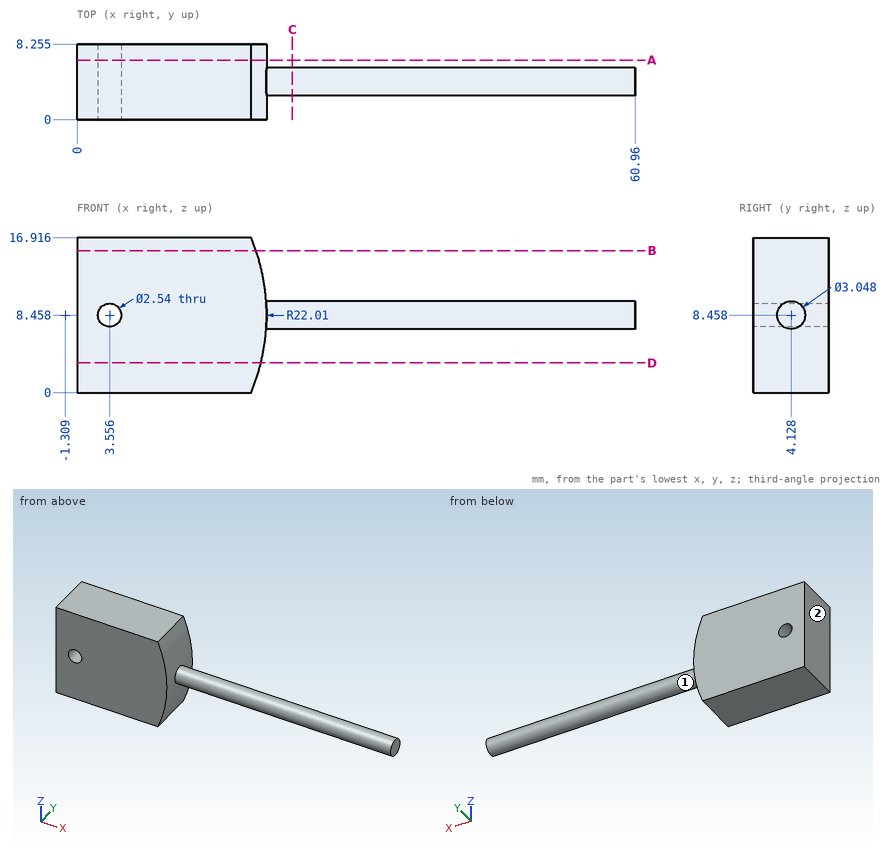
Could you check a few things on this drawing? It's one solid part, dimensions in mm from its lowest x, y, z. A direction names the side the tool comes from. Round coordinates to 2 decimals unless told otherwise and drop trailing zeros. Order: outer loops, then holes, each group sorted by start corner. A loop starts at its lowest first (then second) coordinate and runs counter-clockwise, first axis right, second up. Notation, with made-up numbers: M -8,2 L 7,2 A26 cw 7,19 Z; hole C 59,4 d7. An arc over 180 degrees is marked long. Return JSON: item names as keys, results as strings. Group by question number.
1. If we section it at A-A on y = 6.5: List the corners of the cut face in (x, z) for me (1 decimal), then the cut area to 3 significant figures.
2. If we section it at B-B on z = 15.5: List the corners of the cut face in (x, y) for me (1 decimal), then the cut area to 3 significant figures.
3. On a 3-axis mill with a long thin cutter (end or side, diameter ignored), from which of +Z, -Z, +X, -X, +Y, -Y can I reach the whole of each face in a straight line? I mean the marked faces 1 and 2. Say none if no direction works.
4. If we section it at C-C on x = 23.5: List the corners of the cut face in (y, z) for me (1 decimal).
5. Please list where these lines run through material, in increasing order: probe 1 along Z at (x, y) = (27.5, 4.25); probe 2 along X at (y, z) = (5, 8.75); probe 3 along X at (y, z) = (5, 4) (1 decimal).
6. I'm going to push a flat-ended pin straight in: pin 1 Ø1 at (x, y) = (54, 5.5) entering from -Z. Where does the tip first touch, or does it pass through?
7. If we section it at D-D on z = 3.25: List the corners of the cut face in (x, y) for me (1 decimal).
Reply:
{
 "1": {"outline": "M 0,0 L 19,0 A22 ccw 19,16.9 L 0,16.9 Z; hole C 3.6,8.5 d2.5", "area": "336 mm^2"},
 "2": {"outline": "M 0,0 L 19.5,0 L 19.5,8.3 L 0,8.3 Z", "area": "161 mm^2"},
 "3": {"face 1": "+X", "face 2": "+Z, -Z, -X, +Y, -Y"},
 "4": {"outline": "C 4.1,8.5 d3"},
 "5": {"probe 1": "6.94 to 9.98", "probe 2": "0 to 2.32, 4.79 to 60.96", "probe 3": "0 to 20.2"},
 "6": {"pin 1": "z = 7.21"},
 "7": {"outline": "M 0,0 L 20.1,0 L 20.1,8.3 L 0,8.3 Z"}
}
